Here's how the part is built. I have some questions about the finished solid (model axes, mm). A direction names the side the tool comes from. Give positions to 0.01 mm unless a question says otherwise; leave off trailing zeros. Order: outer loops, then holes, each group sorted by start corner. A loop starts at its lowest first (then second) coordinate and runs counter-clockwise, first axis right, second up. Notation, with made-up numbers: M -11.75,21 L 31.25,21 A11 ccw 31.25,29 Z; hole C 75,62 d2. An arc over 180 degrees is marked long. Use CSV: the item, a comma, the result in double quotes. Start each with the question number.
Autodesk Fusion 360 part; units mm, degrees
sketch "Sketch1" plane through (0, 0, 0) normal (0, 0, 1) x (1, 0, 0) in component "WatchStrapBit"
  line L0 (2, 0) -> (24, 0)
  line L1 (26, -2) -> (26, -5)
  line L2 (24, -7) -> (2, -7)
  line L3 (0, -5) -> (0, -2)
  line L4 (23, -0.8) -> (2.8, -0.8)
  line L5 (0.8, -2.8) -> (0.8, -4.2)
  line L6 (2.8, -6.2) -> (23, -6.2)
  line L7 (25, -4.2) -> (25, -2.8)
  arc A0 (25, -2.8) -> (23, -0.8) centre (23, -2.8) ccw
  arc A1 (23, -6.2) -> (25, -4.2) centre (23, -4.2) ccw
  arc A2 (2.8, -0.8) -> (0.8, -2.8) centre (2.8, -2.8) ccw
  arc A3 (0.8, -4.2) -> (2.8, -6.2) centre (2.8, -4.2) ccw
  arc A4 (2, 0) -> (0, -2) centre (2, -2) ccw
  arc A5 (0, -5) -> (2, -7) centre (2, -5) ccw
  arc A6 (24, -7) -> (26, -5) centre (24, -5) ccw
  arc A7 (26, -2) -> (24, 0) centre (24, -2) ccw
  point P0 (26, 0)
  dimension "d1" = 26
  dimension "d2" = 7
  dimension "d3" = 0.8
  dimension "d4" = 0.8
  dimension "d5" = 1
  dimension "d6" = 0.8
  dimension "d7" = 2
extrude "Extrude1" add sketch "Sketch1" along normal blind 12 in component "WatchStrapBit"
sketch "Sketch2" plane through (0, 0, 0) normal (0, 1, 0) x (-1, 0, 0) in component "WatchStrapBit"
  line L0 (-24, 0) -> (-2, 0)
  line L1 (-2, 0) -> (-2, 12)
  line L2 (-2, 12) -> (-24, 12)
  line L3 (-24, 12) -> (-24, 0)
  line L4 (-24, 0) -> (-2, 0)
  line L5 (-2, 12) -> (-24, 12)
  line L6 (0, 0) -> (-2, 0)
  line L7 (0, 12) -> (-2, 12)
  line L8 (0, 0) -> (0, 12)
  line L9 (-26, 0) -> (-26, 12)
  line L10 (-24, 0) -> (-26, 0)
  line L11 (-24, 12) -> (-26, 12)
  line L12 (0, 0) -> (-26, 0) construction
  line L13 (0, 12) -> (-26, 12) construction
  line L14 (-13, 0) -> (-13, 12) construction
  line L15 (-13, 6) -> (-13, 3.5)
  line L16 (-13, 6) -> (-13, 8.5)
  circle A0 centre (-13, 3.5) radius 0.75
  circle A1 centre (-13, 8.5) radius 0.75
  ellipse E0 centre (-13, 3.5) end of major axis (-13, 2.75) minor radius 1
  line L17 (-13, 4.25) -> (-13, 2.75)
  line L18 (-14, 3.5) -> (-12, 3.5)
  ellipse E1 centre (-13, 8.5) end of major axis (-13, 7.75) minor radius 1
  line L19 (-13, 9.25) -> (-13, 7.75)
  line L20 (-14, 8.5) -> (-12, 8.5)
  point P0 (-13, 0)
  point P1 (-13, 12)
  point P2 (-13, 6)
  dimension "d10" = 2.5
  dimension "d11" = 2.5
  dimension "d12" = 1.5
  dimension "d13" = 1.5
  dimension "d16" = 2
  dimension "d17" = 2
extrude "Extrude2" add sketch "Sketch2" against normal blind 3 contours A0 E0 L18 | L15 A0 L17 L18 | L15 A0 L17 L18 | A0 E0 L18 | A1 E1 L20 | L16 A1 L19 L20 | L16 A1 L19 L20 | A1 E1 L20 | A0 L17 L18 | A0 L17 L18 | A0 E0 L18 | A0 E0 L18 | A1 L19 L20 | A1 L19 L20 | A1 E1 L20 | A1 E1 L20 in component "WatchStrapBit"
component "WatchStrapBit" placed x (1, 0, 0) y (0, 1, 0) z (0, 0, 1) at (0, 0, 0)
equation "d4 = d3"
equation "d6 = d3"
Q1. For P1, Ø1.5, axis at y = -3.5, z = 3.5, coming from the -X side, with a flat end and sliding along its axis, tell me the tip position at first contact or that it passes through.
Q2. Imagine slicing it at C-C, the plane y = -3.75. Please give me the cut outline in (x, z), then the cut area to 3 significant figures.
Q3. Imagine slicing it at A-A, the plane x = 21.5. Please give me the cut outline in (y, z), then the cut area to 3 significant figures.
Q4. For faces 1 (the face through (0.57, -0.6, 5.92)), 2 (the face through (1.37, -1.4, 5.92)), which set-ups out of +Z, -Z, +X, -X, +Y, -Y let a thin tool reach every point of the face, with its end or its side?
Q5. I need wall thicknesses on line 1 (Y direction, x = 19.5, z = 1.5); line 2 (X direction, y = -3.5, z = 2); line 3 (X direction, y = -5, z = 9.25). Which ranges of each line are inside material? Lowest first, please. Write a range as [from, to].
Q6. Imagine slicing it at B-B, the plane z = 2.25. Please give me the cut outline in (x, y), then the cut area to 3 significant figures.
Q7. We'd pull the mould along Y, two halves only. Please class faces 3 (the face through (0, -4, 6)), 4 (the face through (24.4, -1.37, 5.92)), 5 (the face through (25.4, -0.57, 5.92)), 6 (the face through (25.43, -6.4, 5.92)): pulls with the +Y half, pulls with the -Y half, needs draft (parallel to the pull), parting line crosses it, or undercut.
Q8. Imagine slicing it at D-D, the plane y = -1.75. Count the separate pieces of the cut face and the enclosed holes in it, then the cut area to 3 significant figures.
Reply:
1,P1,"stops at x = 0"
2,outline,"M 0,0 L 0.8,0 L 0.8,12 L 0,12 Z; M 25,0 L 26,0 L 26,12 L 25,12 Z"
2,area,"21.6 mm^2"
3,outline,"M -7,0 L -6.2,0 L -6.2,12 L -7,12 Z; M -0.8,0 L 0,0 L 0,12 L -0.8,12 Z"
3,area,"19.2 mm^2"
4,face 1,"+Z, -Z, -X, +Y"
4,face 2,"+Z, -Z"
5,line 1,"y = [-7, -6.2], [-0.8, 0]"
5,line 2,"x = [0, 0.8], [25, 26]"
5,line 3,"x = [0, 0.97], [24.83, 26]"
6,outline,"M 0,-5 A2 ccw 2,-7 L 24,-7 A2 ccw 26,-5 L 26,-2 A2 ccw 24,0 L 2,0 A2 ccw 0,-2 Z; hole M 0.8,-4.2 A2 ccw 2.8,-6.2 L 23,-6.2 A2 ccw 25,-4.2 L 25,-2.8 A2 ccw 23,-0.8 L 2.8,-0.8 A2 ccw 0.8,-2.8 Z"
6,area,"51.3 mm^2"
7,face 3,"needs draft"
7,face 4,"undercut"
7,face 5,"pulls with the +Y half"
7,face 6,"pulls with the -Y half"
8,separate pieces,"4"
8,enclosed holes,"0"
8,area,"33.1 mm^2"
